```python
from build123d import *

# Parameters (mm, degrees)
F1_DEPTH      = 15
F0_R          = 10
F2_DEPTH      = 13
F2_DEPTH_BACK = 15
F0_R_2        = 12.5
F3_DEPTH      = 33
F3_DEPTH_BACK = 15
F0_R_3        = 7.5
F4_DEPTH      = 28
F4_DEPTH_BACK = 10
F5_DEPTH      = 12.5
F5_DEPTH_BACK = 27.5


with BuildPart() as f1:
    # F0 (on Right) → F1 (new body)
    with BuildSketch(Plane.YZ):
        with BuildLine():
            ThreePointArc((-75, 25), (-82.32233, 7.32233), (-100, 0))
            Line((-100, 0), (-10.355339, 0))
            ThreePointArc((-10.355339, 0), (-28.033009, 42.677669), (14.644661, 25))
            ThreePointArc((14.644661, 25), (12.741649, 15.432914), (7.32233, 7.32233))
            Line((7.32233, 7.32233), (83.8967, 83.8967))
            ThreePointArc((83.8967, 83.8967), (62.253682, 85.370134), (64.715921, 106.923061))
            Line((64.715921, 106.923061), (-2.317082, 56.095038))
            ThreePointArc((-2.317082, 56.095038), (-10.881435, 51.564557), (-20.443107, 50))
            Line((-20.443107, 50), (-100, 50))
            ThreePointArc((-100, 50), (-82.32233, 42.67767), (-75, 25))
        make_face()
    extrude(amount=-F1_DEPTH)

    # F0 (on Right) → F2 (join, two sides)
    with BuildSketch(Plane.YZ) as f2_sk:
        with BuildLine():
            ThreePointArc((-100, 50), (-125, 25), (-100, 0))
            ThreePointArc((-100, 0), (-82.32233, 7.32233), (-75, 25))
            ThreePointArc((-75, 25), (-82.32233, 42.67767), (-100, 50))
        make_face()
        with Locations((-100, 25)):
            Circle(F0_R, mode=Mode.SUBTRACT)
    extrude(amount=F2_DEPTH)
    extrude(f2_sk.sketch, amount=-F2_DEPTH_BACK)

    # F0 (on Right) → F3 (join, two sides)
    with BuildSketch(Plane.YZ) as f3_sk:
        with BuildLine():
            ThreePointArc((14.644661, 25), (-28.033009, 42.677669), (-10.355339, 0))
            ThreePointArc((-10.355339, 0), (-0.788253, 1.903012), (7.32233, 7.32233))
            ThreePointArc((7.32233, 7.32233), (12.741649, 15.432914), (14.644661, 25))
        make_face()
        with Locations((-10.355339, 25)):
            Circle(F0_R_2, mode=Mode.SUBTRACT)
    extrude(amount=F3_DEPTH)
    extrude(f3_sk.sketch, amount=-F3_DEPTH_BACK)

    # F0 (on Right) → F4 (join, two sides)
    with BuildSketch(Plane.YZ) as f4_sk:
        with Locations((-10.355339, 25)):
            Circle(F0_R_2)
        with Locations((-10.355339, 25)):
            Circle(F0_R_3, mode=Mode.SUBTRACT)
    extrude(amount=F4_DEPTH)
    extrude(f4_sk.sketch, amount=-F4_DEPTH_BACK)

    # F0 (on Right) → F5 (join, two sides)
    with BuildSketch(Plane.YZ) as f5_sk:
        with BuildLine():
            ThreePointArc((64.715921, 106.923061), (62.253682, 85.370134), (83.8967, 83.8967))
            Line((83.8967, 83.8967), (84.852814, 84.852814))
            ThreePointArc((84.852814, 84.852814), (87.763, 89.544172), (88.778934, 94.97058))
            ThreePointArc((88.778934, 94.97058), (80.45182, 108.404589), (64.715921, 106.923061))
        make_face()
        with Locations((73.778934, 94.97058)):
            Circle(F0_R_3, mode=Mode.SUBTRACT)
    extrude(amount=F5_DEPTH)
    extrude(f5_sk.sketch, amount=-F5_DEPTH_BACK)


solid = f1.part
```
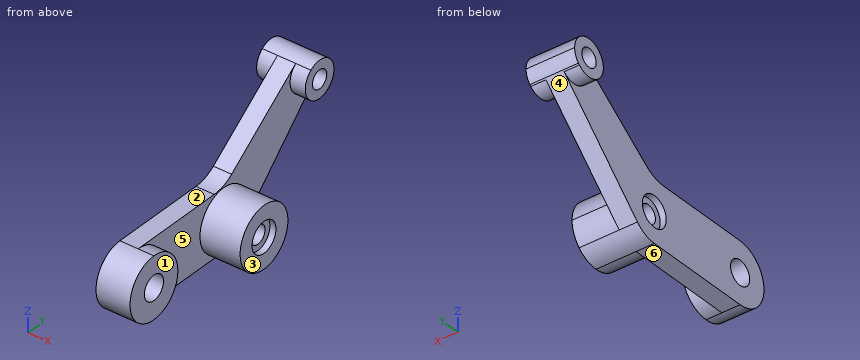
The model under review builds one solid part; all positions refer to its coordinate system, in mm. Face numbers are marked on the shaded views. A direction names the side the tool comes from. Round coordinates to 2 decimals unless told otherwise and drop trailing zeros. Loops run counter-clockwise (first coordinate to the right, second up) from the corner with the lowest first, then second, coordinate; pieces in that order, holes last.
1) Consider section B-B on x = 20.5. State the section outline as (y, z) points.
Values follow:
outline: (-10.36, 0) arc R25 ccw to (7.32, 7.32) arc R25 ccw to (14.64, 25) arc R25 ccw (long way) to start; hole circle Ø15 at (-10.36, 25)
2) Consider section C-C on y = -83. State the section outline as (x, z) points, then the cut area to 3 significant figures.
Values follow:
outline: (-15, 0) - (0, 0) - (0, 6.67) - (13, 6.67) - (13, 43.33) - (0, 43.33) - (0, 50) - (-15, 50) - close
area: 1,230 mm2
3) Wall thickness on line 1 along Z through (x, y) = (11.5, 73); line 2 along X through (y, z) = (49, 94.5); line 3 along Y through (x, z) = (-13.5, 99): over which ranges is each line inside the solid? List them lowest first.
Values follow:
line 1: z = 79.99 to 87.51, 102.43 to 109.95
line 2: x = -15 to 0
line 3: y = 54.27 to 67.45, 80.1 to 88.23
4) Clearance check with flat-ended pins moving along their axes: P1, Ø24, axis at y = 68, z = 100, coming from the +X side; P2, Ø15, axis at y = -99, z = 16, coming from the +X side; P3, Ø2, axis at x = 3, z = 23.5, coming from the +Y side. State where each tip first meets the part, or that it passes through.
Values follow:
P1: stops at x = 12.5
P2: stops at x = 13
P3: stops at y = 14.64
5) Consider section D-D on z = 64.5. State the section outline as (x, y) points, then the cut area to 3 significant figures.
Values follow:
outline: (-15, 8.77) - (0, 8.77) - (0, 64.5) - (-15, 64.5) - close
area: 836 mm2
6) Consider section A-A on x = 2.5. State the section outline as (y, z) points.
Values follow:
outline: (-100, 0) arc R25 ccw to (-75, 25) arc R25 ccw to (-100, 50) arc R25 ccw to start; (-10.36, 0) arc R25 ccw to (7.32, 7.32) arc R25 ccw to (14.64, 25) arc R25 ccw (long way) to start; (64.72, 106.92) arc R15 ccw (long way) to (83.9, 83.9) - (84.85, 84.85) arc R15 ccw to start; hole circle Ø20 at (-100, 25); hole circle Ø15 at (-10.36, 25); hole circle Ø15 at (73.78, 94.97)
7) Tool access review of the marked faces 1, 2 and 3: name each direction out of +Z, -Z, +X, -X, +Y, -Y from which nothing blocks a thin tool from reaching the whole face with its end or side.
Values follow:
face 1: +Z, -Z, +X, -Y
face 2: +Z, +X, -X, -Y
face 3: +Z, -Z, +X, +Y, -Y
8) The part is to be moulded in two halves that separate along Y. For the marked faces 4, 5 and 6, say which applies: pulls with the +Y half, pulls with the -Y half, needs draft (parallel to the pull), parting line crosses it, or undercut.
Values follow:
face 4: pulls with the +Y half
face 5: undercut
face 6: needs draft
